```python
from build123d import *

# Parameters (mm, degrees)
F1_DEPTH = 8
F2_W     = 10
F2_H     = 30
F3_DEPTH = 5
F4_R     = 2
F5_DEPTH = 13.9
F6_DEPTH = 2
F7_R     = 3


with BuildPart() as f1:
    # F0 (on Top) → F1 (new body)
    with BuildSketch(Plane.XY):
        with BuildLine():
            Line((-11, 0), (0, 0))
            ThreePointArc((0, 0), (2.844279, 1.18741), (4, 4.044713))
            Line((4, 4.044713), (4, 26.008084))
            ThreePointArc((4, 26.008084), (2.82557, 28.831284), (0, 30))
            Line((0, 30), (-11, 30))
            Line((-11, 30), (-11, 0))
        make_face()
    extrude(amount=F1_DEPTH)

    # F2 (on face) → F3 (join)
    with BuildSketch(Plane.XY.offset(8)):
        with Locations((-6, 15)):
            Rectangle(F2_W, F2_H)
    extrude(amount=F3_DEPTH)

    # F4 (on face) → F5 (cut)
    with BuildSketch(Plane.XY.offset(13)):
        with Locations((-3.5, 15)):
            Circle(F4_R)
    extrude(amount=-F5_DEPTH, mode=Mode.SUBTRACT)

    # F4 (on face) → F6 (join)
    with BuildSketch(Plane.XY.offset(13)):
        Polygon((-6, 16.5), (-11, 16.5), (-11, 15), (-11, 13.5), (-6, 13.5), (-6, 15), align=None)
    extrude(amount=F6_DEPTH)

    # F7
    f7_edges = [f1.edges().sort_by_distance(p)[0] for p in [
        (-11, 15, 0),
    ]]
    fillet(f7_edges, radius=F7_R)


solid = f1.part
```
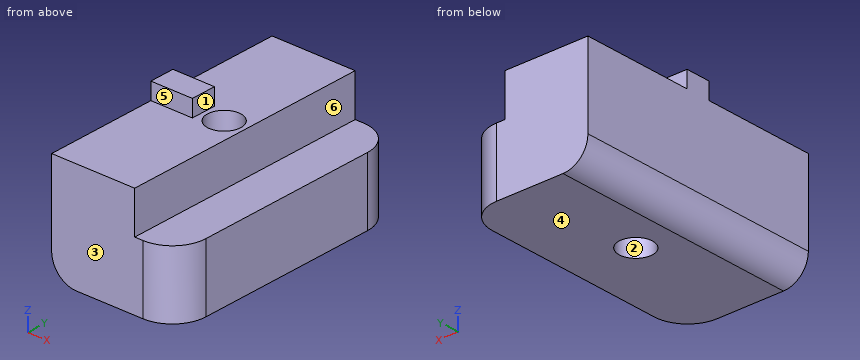
CAD build for the part. Positions are in the model's coordinates, mm. Face numbers are marked on the shaded views. A direction names the side the tool comes from. Round coordinates to 2 decimals unless told otherwise and drop trailing zeros. Order: outer loops, then holes, each group sorted by start corner. A loop starts at its lowest first (then second) coordinate and runs counter-clockwise, first axis right, second up. Notation, with made-up numbers: (57, 41.25) - (92, 41.25) arc R14 cw to (92, 65.25) - close; hole circle Ø10 at (-19.5, 18). An arc over 180 degrees is marked (long way). Answer in a Markdown table with one row per item. Add a question column.
(1) Band-saw the part on D-D on x = -9.5. List the corners of the cut face in (y, z).
(2) Mould opens along Y. For the marked faces 1, 2 and 3 say: +Y half, -Y half, draft (parallel to the pull), parting line (faces both ways), or undercut.
(3) Drop flat-ended pins along their axis: pin 1 Ø0.6 at (y, z) = (15, 14.5) entering from +X; pin 2 Ø4 at (x, z) = (1, 8) entering from -Y; pin 3 Ø2.5 at (y, z) = (16, 11.5) entering from +X; pin 4 Ø0.6 at (x, z) = (-9, 14) entering from -Y. Give the stop position or say it passes through.
(4) Band-saw the part on A-A on y = 15. List the corners of the cut face in (x, z).
(5) Band-saw the part on C-C on x = -3.5. List the corners of the cut face in (y, z).
(6) Band-saw the part on B-B on z = 9.5. List the corners of the cut face in (x, y).
(7) 3-axis set-ups, long thin cutter, end or side, ignore diameter. For the marked faces 4, 5 and 6: which of +Z, -Z, +X, -X, +Y, -Y reach the whole face in a straight line?
(8) Probe L1, parallel to Y at x = -3.5, z = 5; L2, parallel to Z at x = -7.5, y = 19; L3, parallel to Z at x = 2.25, y = 2. List the from-to ranges inside material, lowest first. Write a range as [from, to].
Data:
| question | item | result |
|---|---|---|
| 1 | outline | (0, 0.4) - (30, 0.4) - (30, 13) - (16.5, 13) - (16.5, 15) - (13.5, 15) - (13.5, 13) - (0, 13) - close |
| 2 | face 1 | draft |
| 2 | face 2 | undercut |
| 2 | face 3 | -Y half |
| 3 | pin 1 | stops at x = -6 |
| 3 | pin 2 | stops at y = 0 |
| 3 | pin 3 | stops at x = -1 |
| 3 | pin 4 | stops at y = 13.5 |
| 4 | outline | (-11, 3) arc R3 ccw to (-8, 0) - (-5.5, 0) - (-5.5, 13) - (-6, 13) - (-6, 15) - (-11, 15) - close; (-1.5, 0) - (4, 0) - (4, 8) - (-1, 8) - (-1, 13) - (-1.5, 13) - close |
| 5 | outline | (0, 0) - (13, 0) - (13, 13) - (0, 13) - close; (17, 0) - (30, 0) - (30, 13) - (17, 13) - close |
| 6 | outline | (-11, 0) - (-1, 0) - (-1, 30) - (-11, 30) - close; hole circle Ø4 at (-3.5, 15) |
| 7 | face 4 | -Z, +X, -X, +Y, -Y |
| 7 | face 5 | +Z, +X, -X, -Y |
| 7 | face 6 | +Z, +X, +Y, -Y |
| 8 | L1 | y = [0, 13], [17, 30] |
| 8 | L2 | z = [0, 13] |
| 8 | L3 | z = [0, 8] |
